Geometry: final body of the model. Coordinates: model frame, mm. Face numbers are marked on the shaded views. A direction names the side the tool comes from. Round coordinates to 2 decimals unless told otherwise and drop trailing zeros. Order: outer loops, then holes, each group sorted by start corner. A loop starts at its lowest first (then second) coordinate and runs counter-clockwise, first axis right, second up. Notation, with made-up numbers: (-20.5, 19.25) -> (-16.5, 19.25) arc R32 cw to (-16.5, 48.25) -> close; hole circle Ø7 at (53.25, 15.25). An arc over 180 degrees is marked (long way). Put each result on its own line as item: value.
```python
from build123d import *

# Parameters (mm, degrees)
P_IDAT_VYSUNUT_M1_DEPTH                           = 250
SKICA2_W                                          = 120
SKICA2_H                                          = 210
ODEBRAT_VYSUNUT_M1_DEPTH                          = 100
V_LCOV_ZAHLOUBEN_PRO_M6_ROUBY_S_V_LCO_D           = 6.6
V_LCOV_ZAHLOUBEN_PRO_M6_ROUBY_S_V_LCO_CBORE_D     = 14
V_LCOV_ZAHLOUBEN_PRO_M6_ROUBY_S_V_LCO_CBORE_DEPTH = 115
P_IDAT_VYSUNUT_M2_DEPTH                           = 2
ZKOSEN_1_SIZE                                     = 2


with BuildPart() as part:
    # Skica1 → Přidat vysunutím1 (new body)
    with BuildSketch(Plane.XY):
        with BuildLine():
            Line((0, 0), (0, 105))
            Line((0, 105), (120, 105))
            Line((120, 105), (120, 100))
            ThreePointArc((120, 100), (49.289321881, 70.710678119), (20, 0))
            Line((20, 0), (0, 0))
        make_face()
    extrude(amount=P_IDAT_VYSUNUT_M1_DEPTH)

    # Skica2 → Odebrat vysunutím1 (cut)
    with BuildSketch(Plane.XZ):
        with Locations((60, 125)):
            Rectangle(SKICA2_W, SKICA2_H)
    extrude(amount=-ODEBRAT_VYSUNUT_M1_DEPTH, mode=Mode.SUBTRACT)

    # Válcové zahloubení pro M6 šrouby s válcovou hlavou zaoblenou1 (through all)
    with Locations(Plane(origin=(120, 0, 0), x_dir=(0, 0, -1), z_dir=(1, 0, 0))):
        with Locations((-240, 91), (-240, 15)):
            v_lcov_zahlouben_pro_m6_rouby_s_v_lco = CounterBoreHole(V_LCOV_ZAHLOUBEN_PRO_M6_ROUBY_S_V_LCO_D / 2, V_LCOV_ZAHLOUBEN_PRO_M6_ROUBY_S_V_LCO_CBORE_D / 2, V_LCOV_ZAHLOUBEN_PRO_M6_ROUBY_S_V_LCO_CBORE_DEPTH)

    # Zrcadlit1: Válcové zahloubení pro M6 šrouby s válcovou hlavou zaoblenou1 across plane
    add(v_lcov_zahlouben_pro_m6_rouby_s_v_lco.mirror(Plane.XY.offset(125)), mode=Mode.SUBTRACT)

    # Skica8 → Přidat vysunutím2 (add)
    with BuildSketch(Plane(origin=(0, 105, 0), x_dir=(1, 0, 0), z_dir=(0, 1, 0))):
        Polygon((0, 0), (120, 0), (120, -250), (0, -250), (0, -248.4), (116.8, -248.4), (116.8, -1.6), (0, -1.6), align=None)
    extrude(amount=P_IDAT_VYSUNUT_M2_DEPTH)

    # Zkosení1
    zkosen_1_edges = [part.edges().sort_by_distance(p)[0] for p in [
        (116.8, 107, 125),
    ]]
    chamfer(zkosen_1_edges, length=ZKOSEN_1_SIZE - 0.0001)  # a hair under: the kernel refuses the full size


solid = part.part
```
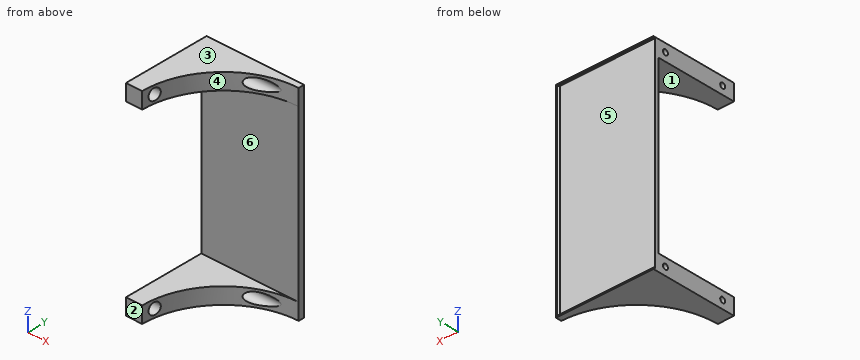
1. Contact query for flat-ended pins moving along their axis: P1, Ø2, axis at x = 46.5, z = 137, coming from the +Y side; P2, Ø8.5, axis at y = 15, z = 10, coming from the +X side; P3, Ø11, axis at y = 13, z = 7, coming from the +X side. Output: stop coordinate, or through.
Ans:
P1: y = 105
P2: x = 5
P3: x = 21.47
2. Cut plane B-B on x = 17.5. Return loops of the section in (y, z).
Ans:
outline: (0, 0) -> (107, 0) -> (107, 1.6) -> (105, 1.6) -> (105, 248.4) -> (107, 248.4) -> (107, 250) -> (0, 250) -> (0, 230) -> (100, 230) -> (100, 20) -> (0, 20) -> close; hole circle Ø14 at (15, 10); hole circle Ø14 at (15, 240); hole circle Ø14 at (91, 10); hole circle Ø14 at (91, 240)
3. Cut plane C-C on z = 240. State how many separate pieces and enclosed holes the cut face has, and give its area (3 significant figures).
Ans:
separate pieces: 3
enclosed holes: 0
area: 3,410 mm²
4. Material intervals for probe 1 along Y at (x, z) = (14, 240); probe 2 along Y at (x, z) = (2, 10); probe 3 along Y at (x, z) = (72.5, 223.5), sorted ascending.
Ans:
probe 1: 0 to 8, 22 to 84, 98 to 105
probe 2: 0 to 11.7, 18.3 to 87.7, 94.3 to 105
probe 3: 100 to 105
5. Cut plane D-D on x = 55.5. Return loops of the section in (y, z).
Ans:
outline: (76.42, 0) -> (107, 0) -> (107, 1.6) -> (105, 1.6) -> (105, 248.4) -> (107, 248.4) -> (107, 250) -> (76.42, 250) -> (76.42, 230) -> (100, 230) -> (100, 20) -> (76.42, 20) -> close; hole circle Ø14 at (91, 10); hole circle Ø14 at (91, 240)
6. Draft query along Z for the marked faces 1, 2 and 3. Return one class per face: +Z half, -Z half, draft (parallel to the pull), parting line (faces both ways), or undercut.
Ans:
face 1: undercut
face 2: draft
face 3: +Z half
7. Set-up query: the marked faces 4, 5 and 6. Return all of +Z, -Z, +X, -X, +Y, -Y with unobstructed straight access to the full face (end or side cutting, diameter ignored); none if empty.
Ans:
face 4: +Z, -Z, +X, -Y
face 5: -X, +Y
face 6: +X, -X, -Y
8. Cut plane A-A on y = 60. Return loops of the section in (x, z).
Ans:
outline: (0, 0) -> (40, 0) -> (40, 20) -> (0, 20) -> close; (0, 230) -> (40, 230) -> (40, 250) -> (0, 250) -> close
